```python
from build123d import *

# Parameters (mm, degrees)
F1_DEPTH = 38.1
F2_R     = 13.716
F3_DEPTH = 50.292
F4_R     = 1.905
F5_DEPTH = 25.4


# Not quite as in the source:
# - a feature names something its author has since deleted; it is built from what else it names


with BuildPart() as f1:
    # F0 (on Top) → F1 (new body)
    with BuildSketch(Plane.XY):
        with BuildLine():
            ThreePointArc((6.1794301228, -15.9926754597), (14.1403209733, -9.6954807912), (17.145, 0))
            ThreePointArc((17.145, 0), (-9.3627294025, 14.3628104191), (-6.9191963412, -15.6868016814))
            ThreePointArc((-6.9191963412, -15.6868016814), (-0.4002539276, -17.1403273537), (6.1794301228, -15.9926754597))
        make_face()
        with BuildLine():
            ThreePointArc((6.1794301228, -15.9926754597), (-0.4002539276, -17.1403273537), (-6.9191963412, -15.6868016814))
            Line((-6.9191963412, -15.6868016814), (-6.9191963412, -23.9002238959))
            Line((-6.9191963412, -23.9002238959), (-16.1695149392, -23.9002238959))
            Line((-16.1695149392, -23.9002238959), (-16.1695149392, -34.5569381251))
            Line((-16.1695149392, -34.5569381251), (17.6482256417, -34.0591232702))
            Line((17.6482256417, -34.0591232702), (17.4986813217, -23.9002238959))
            Line((17.4986813217, -23.9002238959), (6.1794301228, -23.9002238959))
            Line((6.1794301228, -23.9002238959), (6.1794301228, -21.5747152004))
            Line((6.1794301228, -21.5747152004), (6.1794301228, -15.9926754597))
        make_face()
    extrude(amount=F1_DEPTH)

    # F2 (on face) → F3 (cut)
    with BuildSketch(Plane.XY.offset(38.1)):
        Circle(F2_R)
    extrude(amount=-F3_DEPTH, mode=Mode.SUBTRACT)

    # F4 (on face) → F5 (cut)
    with BuildSketch(Plane(origin=(0, -23.9002238959, 0), x_dir=(-1, 0, 0), z_dir=(0, 1, 0))):
        with Locations((11.3007957116, 17.8492013365)):
            Circle(F4_R)
    extrude(amount=-F5_DEPTH, mode=Mode.SUBTRACT)


solid = f1.part
```
Here's how the part is built. I have some questions about the finished solid (model axes, mm). A direction names the side the tool comes from. Give positions to 0.01 mm unless a question says otherwise; leave off trailing zeros. Order: outer loops, then holes, each group sorted by start corner. A loop starts at its lowest first (then second) coordinate and runs counter-clockwise, first axis right, second up. Notation, with made-up numbers: (14.5, -2.75) -> (53.5, -2.75) arc R29 cw to (53.5, 26.25) -> close; hole circle Ø4 at (59, -24). An arc over 180 degrees is marked (long way). Use CSV: the item, a comma, the result in double quotes. Start each with the question number.
Item 1: I'm going to push flat-ended pins straight in: P1, Ø1, axis at x = 14, y = 2, coming from the -Z side; P2, Ø3.5, axis at x = -11.3, z = 17.85, coming from the +Y side; P3, Ø1, axis at y = -14.5, z = 8, coming from the +X side; P4, Ø5.5, axis at x = 10, z = 14, coming from the +Y side. Where does each tip first touch, or does it pass through?
Item 2: On a 3-axis mill with a long thin cutter (end or side, diameter ignored), from which of +Z, -Z, +X, -X, +Y, -Y can I reach the whole of each face in a straight line? I mean faces 1 (the cylindrical face through (1.06, 17.112, 18.783)), 2 (the flat face through (-14, -23.9, 19)), 3 (the flat face through (0, -14, 0)), 4 (the flat face through (12, -23.9, 19)), 5 (the flat face through (-16.17, -29, 19)). Say none if no direction works.
Item 3: If I drill on probe 1 along Y at (x, z) = (9, 8.5); probe 2 along Y at (x, z) = (-8.5, 25.5); probe 3 along Y at (x, z) = (-5.5, 17), over which ranges is the centre line in solid material (lowest first)? Write a range as [from, to].
Item 4: Suppose I cut it at C-C (x = 7). List the corners of the cut face in (y, z) for me.
Item 5: Suppose I cut it at B-B (x = -11). List the corners of the cut face in (y, z) for me, and give its area (3 significant figures).
Item 6: Thinking about a two-plate mould opening in X: for faces 6 (the cylindrical face through (-10.89, -29.13, 15.99)), 7 (the flat face through (0, -14, 38.1)), 8 (the flat face through (-6.919, -20, 19)), which applies, pulls with the +X half, pulls with the -X half, needs draft (parallel to the pull), parting line crosses it, or undercut?
Item 7: Suppose I cut it at D-D (z = 28). List the corners of the cut face in (x, y) for me (3 decimals), and give its area (3 significant figures).
Item 8: Suppose I cut it at A-A (y = 0). List the corners of the cut face in (x, z) for me (3 decimals), and give its area (3 significant figures).
Answer block:
1,P1,"stops at z = 0"
1,P2,"stops at y = 14.24"
1,P3,"stops at x = 9.9"
1,P4,"stops at y = 15.54"
2,face 1,"+Z, -Z"
2,face 2,"+Z, -Z, -X"
2,face 3,"-Z, +X, -X, +Y, -Y"
2,face 4,"+Z, -Z, +X"
2,face 5,"+Z, -Z, -X, -Y"
3,probe 1,"y = [-34.19, -23.9], [-14.59, -10.35], [10.35, 14.59]"
3,probe 2,"y = [-34.44, -23.9], [-14.89, -10.76], [10.76, 14.89]"
3,probe 3,"y = [-34.4, -12.56], [12.56, 16.24]"
4,outline,"(-34.22, 0) -> (-23.9, 0) -> (-23.9, 38.1) -> (-34.22, 38.1) -> close; (-15.65, 0) -> (-11.8, 0) -> (-11.8, 38.1) -> (-15.65, 38.1) -> close; (11.8, 0) -> (15.65, 0) -> (15.65, 38.1) -> (11.8, 38.1) -> close"
5,outline,"(-34.48, 0) -> (-23.9, 0) -> (-23.9, 15.97) -> (-34.48, 15.97) -> close; (-34.48, 19.73) -> (-23.9, 19.73) -> (-23.9, 38.1) -> (-34.48, 38.1) -> close; (-13.15, 0) -> (-8.19, 0) -> (-8.19, 38.1) -> (-13.15, 38.1) -> close; (8.19, 0) -> (13.15, 0) -> (13.15, 38.1) -> (8.19, 38.1) -> close"
5,area,"741 mm^2"
6,face 6,"undercut"
6,face 7,"needs draft"
6,face 8,"pulls with the -X half"
7,outline,"(-16.17, -34.557) -> (17.648, -34.059) -> (17.499, -23.9) -> (6.179, -23.9) -> (6.179, -15.993) arc R17.145 ccw (long way) to (-6.919, -15.687) -> (-6.919, -23.9) -> (-16.17, -23.9) -> close; hole circle Ø27.432 at (0, 0)"
7,area,"778 mm^2"
8,outline,"(-17.145, 0) -> (-13.716, 0) -> (-13.716, 38.1) -> (-17.145, 38.1) -> close; (13.716, 0) -> (17.145, 0) -> (17.145, 38.1) -> (13.716, 38.1) -> close"
8,area,"261 mm^2"
